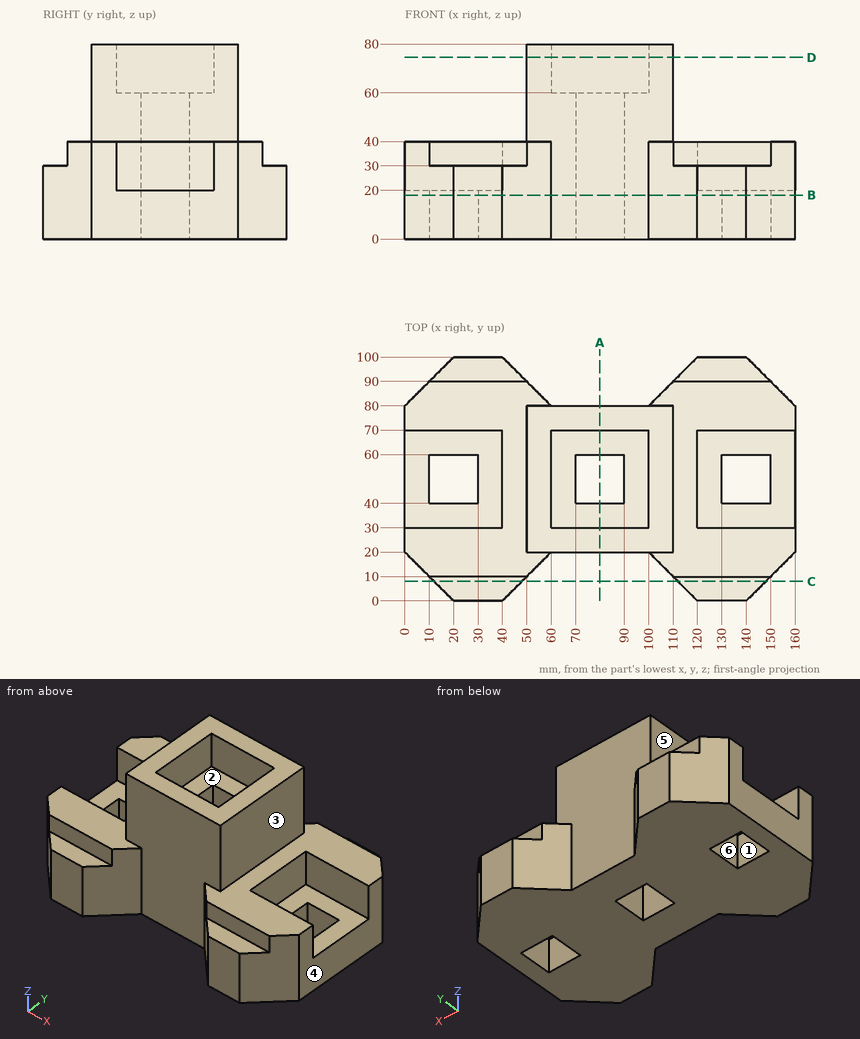
Source: three-view drawing plus pictorial views. Frame: mm from the lowest corner of the part. A direction names the side the tool comes from. Give positions to 0.01 mm unless a question says otherwise; leave off trailing zeros. Order: outer loops, then holes, each group sorted by start corner. A loop starts at its lowest first (then second) coordinate and runs counter-clockwise, first axis right, second up. Notation, with made-up numbers: (76, 0.5) -> (99, 0.5) arc R14 cw to (99, 9.5) -> close; hole circle Ø10 at (70, 55). An arc over 180 degrees is marked (long way). Use a Markdown table: item, result.
Q1. Section C-C (y = 8). Return the cut outline in (x, z).
A:
| item | result |
|---|---|
| outline | (12, 0) -> (48, 0) -> (48, 30) -> (12, 30) -> close; (112, 0) -> (148, 0) -> (148, 30) -> (112, 30) -> close |
Q2. Pull-direction query (X, two-part tool) for the marked faces 4, 5 and 6; classes: +X half, -X half, draft (parallel to the pull), parting line (faces both ways), or undercut.
A:
| item | result |
|---|---|
| face 4 | +X half |
| face 5 | -X half |
| face 6 | undercut |
Q3. Section A-A (x = 80). Return the cut outline in (y, z).
A:
| item | result |
|---|---|
| outline | (20, 0) -> (40, 0) -> (40, 60) -> (30, 60) -> (30, 80) -> (20, 80) -> close; (60, 0) -> (80, 0) -> (80, 80) -> (70, 80) -> (70, 60) -> (60, 60) -> close |
Q4. Section B-B (z = 18). Return the cut outline in (x, y).
A:
| item | result |
|---|---|
| outline | (0, 20) -> (20, 0) -> (40, 0) -> (60, 20) -> (100, 20) -> (120, 0) -> (140, 0) -> (160, 20) -> (160, 80) -> (140, 100) -> (120, 100) -> (100, 80) -> (60, 80) -> (40, 100) -> (20, 100) -> (0, 80) -> close; hole (10, 40) -> (30, 40) -> (30, 60) -> (10, 60) -> close; hole (70, 40) -> (90, 40) -> (90, 60) -> (70, 60) -> close; hole (130, 40) -> (150, 40) -> (150, 60) -> (130, 60) -> close |
Q5. Material intervals for line 1 (X direction, y = 44, z = 8.5); line 2 (Y direction, x = 71, z = 58); line 3 (Y direction, x = 122.5, z = 24), sorted ascending. Write a range as [from, to].
A:
| item | result |
|---|---|
| line 1 | [0, 10], [30, 70], [90, 130], [150, 160] |
| line 2 | [20, 40], [60, 80] |
| line 3 | [0, 30], [70, 100] |
Q6. Access query for the marked faces 1, 2 and 3. Directions: +Z, -Z, +X, -X, +Y, -Y. A direction counts if a zero-diameter tool reaches every point of the face in a straight line with its end or side. Return the directions, or none.
A:
| item | result |
|---|---|
| face 1 | +Z, -Z |
| face 2 | +Z |
| face 3 | +Z, +X, +Y, -Y |
Q7. First-contact query: P1, Ø16, axis at y = 41.5, z = 32.5, coming from the +X side; P2, Ø11, axis at x = 29.5, z = 37.5, coming from the +Y side; P3, Ø4, axis at x = 62.5, y = 21.5, coming from the -Z side; P4, Ø3, axis at x = 46.5, y = 30.5, coming from the +Z side. Flat tips, straight axial feed; report the tip coordinate or a pass-through.
A:
| item | result |
|---|---|
| P1 | x = 120 |
| P2 | y = 90 |
| P3 | z = 0 |
| P4 | z = 40 |
Q8. Section D-D (z = 74.5). Return the cut outline in (x, y).
A:
| item | result |
|---|---|
| outline | (50, 20) -> (110, 20) -> (110, 80) -> (50, 80) -> close; hole (60, 30) -> (100, 30) -> (100, 70) -> (60, 70) -> close |
